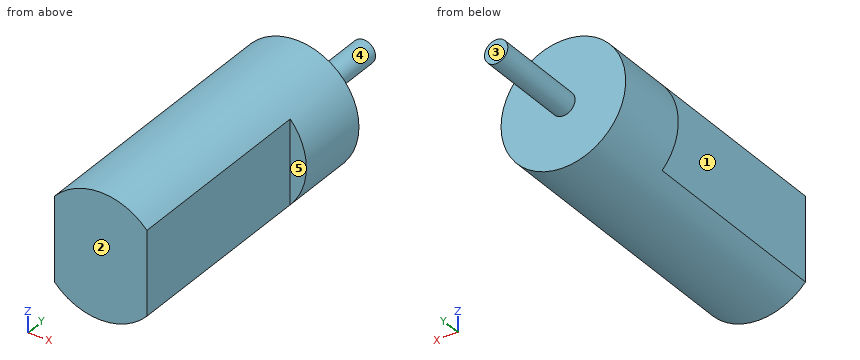
```python
from build123d import *

# Parameters (mm, degrees)
SKETCH1_R           = 8
BOSS_EXTRUDE1_DEPTH = 36.4236
CUT_EXTRUDE1_DEPTH  = 26.6446
SKETCH3_R           = 1.5
BOSS_EXTRUDE2_DEPTH = 12.4968


with BuildPart() as part:
    # Sketch1 → Boss-Extrude1 (new body)
    with BuildSketch(Plane(origin=(0, 0, 0), x_dir=(1, 0, 0), z_dir=(0, 1, 0))):
        Circle(SKETCH1_R)
    extrude(amount=BOSS_EXTRUDE1_DEPTH)

    # Sketch2 → Cut-Extrude1 (cut)
    with BuildSketch(Plane.XZ):
        with BuildLine():
            Line((5.9309, 5.368838346), (5.9309, -5.368838346))
            ThreePointArc((5.9309, -5.368838346), (8, 0), (5.9309, 5.368838346))
        make_face()
        with BuildLine():
            Line((-5.9309, 5.368838346), (-5.9309, -5.368838346))
            ThreePointArc((-5.9309, -5.368838346), (-8, 0), (-5.9309, 5.368838346))
        make_face()
    extrude(amount=-CUT_EXTRUDE1_DEPTH, mode=Mode.SUBTRACT)

    # Sketch3 → Boss-Extrude2 (add)
    with BuildSketch(Plane(origin=(0, 36.4236, 0), x_dir=(1, 0, 0), z_dir=(0, 1, 0))):
        Circle(SKETCH3_R)
    extrude(amount=BOSS_EXTRUDE2_DEPTH)


solid = part.part
```
Model file for the job. Use its own axes, mm. Face numbers are marked on the shaded views. A direction names the side the tool comes from. Round coordinates to 2 decimals unless told otherwise and drop trailing zeros. Write each loop counter-clockwise with the first axis right and the second up, starting at its lowest first coordinate (ties: lowest second). Pieces come first, ordered by that corner, then holes. Notation, with made-up numbers: (-24.5, 1.25) - (-1.5, 1.25) arc R27 ccw to (-1.5, 26.25) - close; hole circle Ø9 at (-10, 52.25). An arc over 180 degrees is marked (long way). Use CSV: the item, a comma, the result in double quotes. Start each with the question number.
Item 1: Pin check, flat tips, straight feed: P1, Ø6, axis at x = -3.5, y = 42, coming from the -Z side; P2, Ø1, axis at x = 5, y = 26.5, coming from the -Z side; P3, Ø4, axis at y = 18, z = -5, coming from the -X side. Stop position of each tip, or through.
Item 2: Drill centre lines: L1, parallel to X at y = 11, z = 1; L2, parallel to Y at x = -4.25, z = -3; L3, parallel to Y at x = 7, z = 2. Where is each one in solid material? Low to high. Write a range as [from, to].
Item 3: Band-saw the part on D-D (z = -2.5). Write the cut outline in (x, y), and give its area (3 significant figures).
Item 4: Band-saw the part on B-B (x = 0). Write the cut outline in (y, z).
Item 5: Tool access for the marked faces 1, 2, 3, 4 and 5: list every direction of +Z, -Z, +X, -X, +Y, -Y with a clear straight run to the whole face (end or side of a thin tool).
Item 6: Band-saw the part on A-A (z = 0). Write the cut outline in (x, y).
Item 7: Band-saw the part on C-C (y = 28). Write the cut outline in (x, z).
Checked values:
1,P1,"stops at z = -1.41"
1,P2,"stops at z = -6.61"
1,P3,"stops at x = -5.93"
2,L1,"x = [-5.93, 5.93]"
2,L2,"y = [0, 36.42]"
2,L3,"y = [26.64, 36.42]"
3,outline,"(-7.6, 26.64) - (-5.93, 26.64) - (-5.93, 0) - (5.93, 0) - (5.93, 26.64) - (7.6, 26.64) - (7.6, 36.42) - (-7.6, 36.42) - close"
3,area,"465 mm²"
4,outline,"(0, -8) - (36.42, -8) - (36.42, -1.5) - (48.92, -1.5) - (48.92, 1.5) - (36.42, 1.5) - (36.42, 8) - (0, 8) - close"
5,face 1,"+Z, -Z, -X, -Y"
5,face 2,"+Z, -Z, +X, -X, -Y"
5,face 3,"+Z, -Z, +X, -X, +Y"
5,face 4,"+Y"
5,face 5,"+Z, -Z, +X, -Y"
6,outline,"(-8, 26.64) - (-5.93, 26.64) - (-5.93, 0) - (5.93, 0) - (5.93, 26.64) - (8, 26.64) - (8, 36.42) - (1.5, 36.42) - (1.5, 48.92) - (-1.5, 48.92) - (-1.5, 36.42) - (-8, 36.42) - close"
7,outline,"circle Ø16 at (0, 0)"
